Verification items for this drawing (mm, ordinates from the low corner). A direction names the side the tool comes from. Coordinates: 2 decimals unless noted, no trailing zeros. Loops run counter-clockwise (first coordinate to the right, second up) from the corner with the lowest first, then second, coordinate; pieces in that order, holes last. Notation, with made-up numbers: M -7,15.5 L 3,15.5 A21 ccw 3,23.5 Z; hole C -21.75,33.25 d8. An arc over 180 degrees is marked long. Return JSON: item names as keys, results as strings.
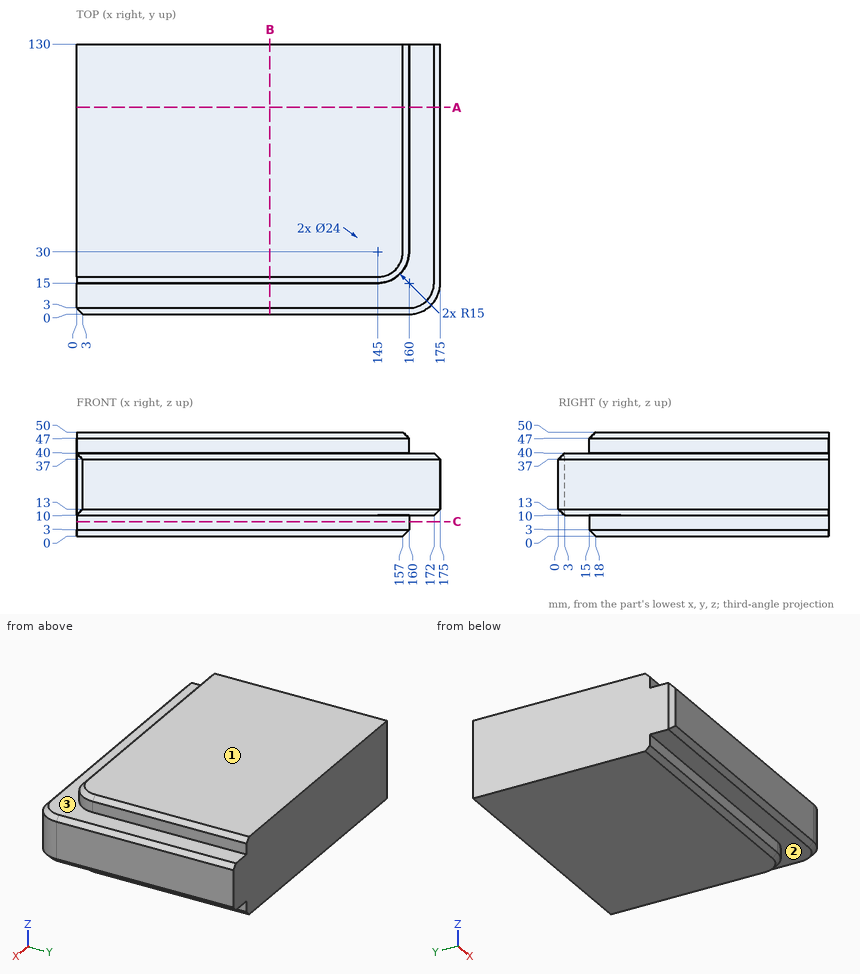
1) Section check A-A on y = 99.5. Record the cut outline in (x, z).
Answers:
{"outline": "M 0,0 L 157,0 L 160,3 L 160,10 L 172,10 L 175,13 L 175,37 L 172,40 L 160,40 L 160,47 L 157,50 L 0,50 Z"}
2) Set-up check for the marked faces 1, 2 and 3: record each of +Z, -Z, +X, -X, +Y, -Y from which the full face is reachable in a straight line by a thin tool's end or side.
Answers:
{"face 1": "+Z, +X, -X, +Y, -Y", "face 2": "-Z, +X, -Y", "face 3": "+Z, +X, -Y"}
3) Section check C-C on z = 7. Record the cut outline in (x, y), then the cut area to 3 significant figures.
Answers:
{"outline": "M 0,15 L 145,15 A15 ccw 160,30 L 160,130 L 0,130 Z", "area": "18,400 mm²"}
4) Section check B-B on x = 93. Record the cut outline in (y, z).
Answers:
{"outline": "M 0,13 L 3,10 L 15,10 L 15,3 L 18,0 L 130,0 L 130,50 L 18,50 L 15,47 L 15,40 L 3,40 L 0,37 Z"}
5) Go/stop test with flat-tipped pins: pin 1 Ø5.5 at (y, z) = (69.5, 43.5) entering from +X; pin 2 Ø5 at (y, z) = (21, 11) entering from -X; pin 3 Ø7.5 at (y, z) = (72.5, 7) entering from +X; pin 4 Ø3.5 at (x, z) = (44.5, 5.5) entering from -Y. Record where each tip stops, or that it passes through.
Answers:
{"pin 1": "x = 160", "pin 2": "x = 0", "pin 3": "x = 172.75", "pin 4": "y = 15"}
6) Scan lines: line 1 along X through (y, z) = (68.5, 6.5); line 2 along Z through (x, y) = (27, 11); line 3 along Y through (x, z) = (31.5, 8). Record each from-to range of solid material in increasing order. Write a range as [from, to].
Answers:
{"line 1": "[0, 160]", "line 2": "[10, 40]", "line 3": "[15, 130]"}
